```python
from build123d import *

# Parameters (mm, degrees)
SKETCH1_W           = 30
SKETCH1_H           = 19
BOSS_EXTRUDE1_DEPTH = 1
SKETCH2_W           = 13.222286428
SKETCH2_H           = 10.81458632
BOSS_EXTRUDE2_DEPTH = 4
SKETCH3_R           = 1
CUT_EXTRUDE1_DEPTH  = 36.73513677


with BuildPart() as part:
    # Sketch1 → Boss-Extrude1 (new body)
    with BuildSketch(Plane(origin=(0, 0, 0), x_dir=(1, 0, 0), z_dir=(0, 1, 0))):
        with Locations((15, 9.5)):
            Rectangle(SKETCH1_W, SKETCH1_H)
    extrude(amount=BOSS_EXTRUDE1_DEPTH)

    # Sketch2 → Boss-Extrude2 (add)
    with BuildSketch(Plane(origin=(0, 1, 0), x_dir=(1, 0, 0), z_dir=(0, 1, 0))):
        with Locations((15.872791289, 11.877603857)):
            Rectangle(SKETCH2_W, SKETCH2_H)
    extrude(amount=BOSS_EXTRUDE2_DEPTH)

    # Sketch3 → Cut-Extrude1 (cut, through all)
    with BuildSketch(Plane(origin=(0, 1, 0), x_dir=(1, 0, 0), z_dir=(0, 1, 0))):
        with Locations(Location((1.396494389, 17.886822044, 0), (0, 0, 270))):
            Circle(SKETCH3_R)
        with Locations(Location((1.396494389, 15.519250271, 0), (0, 0, 270))):
            Circle(SKETCH3_R)
        with Locations(Location((1.396494389, 3.520878065, 0), (0, 0, 270))):
            Circle(SKETCH3_R)
        with Locations(Location((1.396494389, 1.273691297, 0), (0, 0, 270))):
            Circle(SKETCH3_R)
        with Locations(Location((28.603505611, 1.634846313, 0), (0, 0, 270))):
            Circle(SKETCH3_R)
        with Locations(Location((28.603505611, 4.062610589, 0), (0, 0, 270))):
            Circle(SKETCH3_R)
        with Locations(Location((28.603505611, 17.886822044, 0), (0, 0, 270))):
            Circle(SKETCH3_R)
        with Locations(Location((28.603505611, 15.519250271, 0), (0, 0, 270))):
            Circle(SKETCH3_R)
    extrude(amount=-CUT_EXTRUDE1_DEPTH, mode=Mode.SUBTRACT)


solid = part.part
```
Verification items for the finished model (mm, model axes). A direction names the side the tool comes from. Give positions to 0.01 mm unless a question says otherwise; leave off trailing zeros. Write each loop counter-clockwise with the first axis right and the second up, starting at its lowest first coordinate (ties: lowest second). Pieces come first, ordered by that corner, then holes. Notation, with made-up numbers: M 6,-40 L 43,-40 A15 cw 43,-25 Z; hole C 83.25,69 d10. An arc over 180 degrees is marked long. One line per question, with ' | ' between items.
1) Section check A-A on x = 14.5. Enter the section's corners in (y, z), plus the area to 3 significant figures.
Result:
outline: M 0,-19 L 1,-19 L 1,-17.28 L 5,-17.28 L 5,-6.47 L 1,-6.47 L 1,0 L 0,0 Z | area: 62.3 mm2
2) Thickness scan on line 1 along X through (y, z) = (0.2, -3.5); line 2 along X through (y, z) = (2.6, -15); line 3 along Z through (x, y) = (14.25, 2.25). Record the ranges inside material, lowest first. Write a range as [from, to].
Result:
line 1: x = [0, 0.4], [2.4, 27.78], [29.43, 30] | line 2: x = [9.26, 22.48] | line 3: z = [-17.28, -6.47]
3) Section check D-D on y = 3.15. Enter the section's corners in (x, z), plus the area to 3 significant figures.
Result:
outline: M 9.26,-17.28 L 22.48,-17.28 L 22.48,-6.47 L 9.26,-6.47 Z | area: 143 mm2
4) Set-up check for faces 1 (the cylindrical face through (29.45, 0.51, -3.53)), 2 (the flat face through (9.262, 3, -12)), 3 (the flat face through (16, 3, -6.47)), 4 (the flat face through (22.484, 3, -12)), 5 (the flat face through (16, 3, -17.285)): record each of +Z, -Z, +X, -X, +Y, -Y from which the full face is reachable in a straight line by a thin tool's end or side.
Result:
face 1: +Y, -Y | face 2: +Z, -Z, -X, +Y | face 3: +Z, +X, -X, +Y | face 4: +Z, -Z, +X, +Y | face 5: -Z, +X, -X, +Y
5) Section check B-B on y = 0.55. State how many separate pieces and enclosed holes the cut face has, plus the area to 3 significant figures.
Result:
separate pieces: 1 | enclosed holes: 8 | area: 545 mm2
6) Gauge pin test, flat ends, axial feed: pin 1 Ø2.5 at (x, z) = (1.4, -3.52) entering from +Y; pin 2 Ø3 at (y, z) = (3.5, -14) entering from -X; pin 3 Ø1.2 at (x, y) = (14.5, 3) entering from +Z. Record the tip position at first contact, or that the pin passes through.
Result:
pin 1: stops at y = 1 | pin 2: stops at x = 9.26 | pin 3: stops at z = -6.47
7) Mould release check, pull along X, two halves, no side actions. Record for faces 6 (the flat face through (14.8, 0.5, 0)), 7 (the flat face through (0, 0.5, -9.4)), 8 (the cylindrical face through (0.51, 0.51, -0.81)), 9 (the flat face through (30, 0.5, -9.4)): released by +X, released by -X, zero draft, split by the parting line, or undercut.
Result:
face 6: zero draft | face 7: released by -X | face 8: undercut | face 9: released by +X
8) Section check C-C on z = -14. Enter the section's corners in (x, y).
Result:
outline: M 0,0 L 30,0 L 30,1 L 22.48,1 L 22.48,5 L 9.26,5 L 9.26,1 L 0,1 Z
